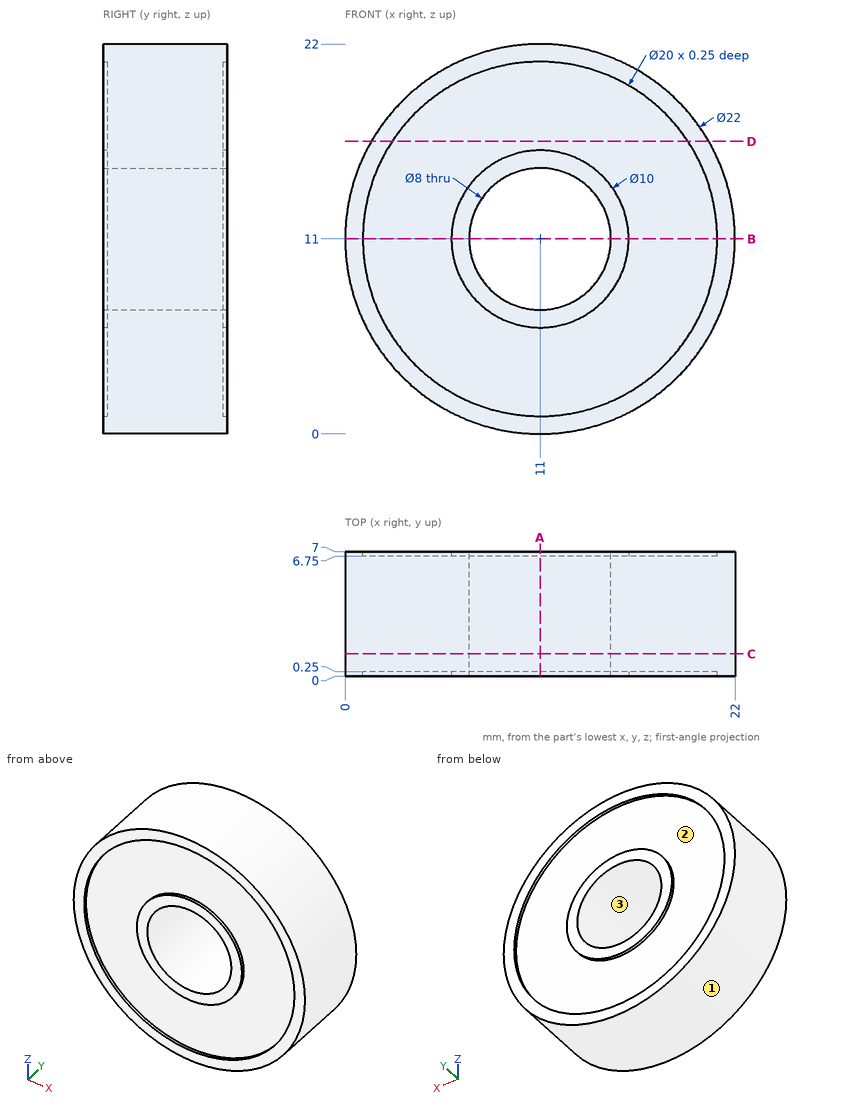
Design review of the part shown in the three views and the two pictorial views. Dimensions are in mm from the part's minimum x, y and z. Coordinates: 2 decimals unless noted, no trailing zeros. Loops run counter-clockwise (first coordinate to the right, second up) from the corner with the lowest first, then second, coordinate; pieces in that order, holes last.
(1) Consider section A-A, the plane x = 11. Give the boundary of the cut face in (y, z).
Determined:
outline: (0, 0) - (7, 0) - (7, 1) - (6.75, 1) - (6.75, 6) - (7, 6) - (7, 7) - (0, 7) - (0, 6) - (0.25, 6) - (0.25, 1) - (0, 1) - close; (0, 15) - (7, 15) - (7, 16) - (6.75, 16) - (6.75, 21) - (7, 21) - (7, 22) - (0, 22) - (0, 21) - (0.25, 21) - (0.25, 16) - (0, 16) - close
(2) Draft analysis for pull direction Z (two halves, no side actions). For the marked faces 1, 2 and 3, state which applies: +Z half, -Z half, draft (parallel to the pull), parting line (faces both ways), or undercut.
Determined:
face 1: parting line
face 2: undercut
face 3: undercut
(3) Consider section C-C, the plane y = 1.25. Give the boundary of the cut face in (x, z), plus the area to 3 significant figures.
Determined:
outline: circle Ø22 at (11, 11); hole circle Ø8 at (11, 11)
area: 330 mm2
(4) Consider section B-B, the plane z = 11. Give the boundary of the cut face in (x, y), plus the area to 3 significant figures.
Determined:
outline: (0, 0) - (1, 0) - (1, 0.25) - (6, 0.25) - (6, 0) - (7, 0) - (7, 7) - (6, 7) - (6, 6.75) - (1, 6.75) - (1, 7) - (0, 7) - close; (15, 0) - (16, 0) - (16, 0.25) - (21, 0.25) - (21, 0) - (22, 0) - (22, 7) - (21, 7) - (21, 6.75) - (16, 6.75) - (16, 7) - (15, 7) - close
area: 93.0 mm2
(5) Consider section D-D, the plane z = 16.5. Give the boundary of the cut face in (x, y).
Determined:
outline: (1.47, 0) - (2.65, 0) - (2.65, 0.25) - (19.35, 0.25) - (19.35, 0) - (20.53, 0) - (20.53, 7) - (19.35, 7) - (19.35, 6.75) - (2.65, 6.75) - (2.65, 7) - (1.47, 7) - close
(6) Insertion check: P1, Ø2, axis at y = 5.5, z = 13.5, coming from the -X side. The pin has a flat end and moves straight along its axis. Give the tip position at first contact, or say it passes through.
Determined:
P1: stops at x = 0.1
(7) Wall thickness on L1, parallel to Z at x = 11, y = 0.2; L2, parallel to Z at x = 11, y = 4.75; L3, parallel to Y at x = 15, z = 2.5: over which ranges is each line inside the solid? List them lowest first.
Determined:
L1: z = 0 to 1, 6 to 7, 15 to 16, 21 to 22
L2: z = 0 to 7, 15 to 22
L3: y = 0.25 to 6.75
